Input: part model. Units: mm. Frame: model coordinates. A direction names the side the tool comes from. Round coordinates to 2 decimals unless told otherwise and drop trailing zeros. Order: outer loops, then holes, each group sorted by start corner. A loop starts at its lowest first (then second) coordinate and runs counter-clockwise, first axis right, second up. Notation, with made-up numbers: (30.25, -9.75) -> (60.25, -9.75) arc R13 cw to (60.25, 5.25) -> close; hole circle Ø3 at (83, 24.25). An arc over 180 degrees is marked (long way). Use a Markdown table: item, result.
from build123d import *

# Parameters (mm, degrees)
REVOLVE1_ANGLE      = 180
SKETCH4_R           = 41.29501491
BOSS_EXTRUDE1_DEPTH = 7
SKETCH5_R           = 34.5
BOSS_EXTRUDE2_DEPTH = 12
SKETCH6_R           = 39
BOSS_EXTRUDE4_DEPTH = 4
SKETCH7_R           = 30
CUT_EXTRUDE1_DEPTH  = 24
CUT_EXTRUDE2_DEPTH  = 10


with BuildPart() as part:
    # Sketch1 → Revolve1 (revolve)
    with BuildSketch(Plane(origin=(0, 0, 0), x_dir=(1, 0, 0), z_dir=(0, 1, 0))):
        with BuildLine():
            Line((1.220496419, 44.983445716), (-1.220496419, -44.983445716))
            ThreePointArc((-1.220496419, -44.983445716), (44.983445716, -1.220496419), (1.220496419, 44.983445716))
        make_face()
    revolve(axis=Axis((1.220496419, 0, -44.983445716), (-0.027122143, 0, 0.999632127)), revolution_arc=REVOLVE1_ANGLE)

    # Sketch2 → Cut-Revolve1 (revolve, cut)
    with BuildSketch(Plane.XZ):
        with BuildLine():
            Line((39.984553657, 1.111516454), (-39.984553657, -1.111516454))
            ThreePointArc((-39.984553657, -1.111516454), (-1.111516454, 39.984553657), (39.984553657, 1.111516454))
        make_face()
    revolve(axis=Axis((39.984553657, 0, 1.111516454), (-0.999613841, 0, -0.027787911)), mode=Mode.SUBTRACT)

    # Sketch4 → Boss-Extrude1 (add)
    with BuildSketch(Plane.XZ):
        Circle(SKETCH4_R)
    extrude(amount=-BOSS_EXTRUDE1_DEPTH)

    # Sketch5 → Boss-Extrude2 (add)
    with BuildSketch(Plane.XZ):
        Circle(SKETCH5_R)
    extrude(amount=BOSS_EXTRUDE2_DEPTH)

    # Sketch6 → Boss-Extrude4 (add)
    with BuildSketch(Plane.XZ.offset(12)):
        Circle(SKETCH6_R)
    extrude(amount=-BOSS_EXTRUDE4_DEPTH)

    # Sketch7 → Cut-Extrude1 (cut)
    with BuildSketch(Plane.XZ.offset(12)):
        Circle(SKETCH7_R)
    extrude(amount=-CUT_EXTRUDE1_DEPTH, mode=Mode.SUBTRACT)

    # Sketch8 → Cut-Extrude2 (cut)
    with BuildSketch(Plane.XZ.offset(12)):
        with BuildLine():
            ThreePointArc((37.671107225, 10.093942759), (19.5, 33.774990748), (-10.093942759, 37.671107225))
            Line((-10.093942759, 37.671107225), (-9.058666579, 33.80740392))
            ThreePointArc((-9.058666579, 33.80740392), (17.5, 30.310889132), (33.80740392, 9.058666579))
            Line((33.80740392, 9.058666579), (37.671107225, 10.093942759))
        make_face()
        with BuildLine():
            ThreePointArc((-10.093942759, -37.671107225), (19.5, -33.774990748), (37.671107225, -10.093942759))
            Line((37.671107225, -10.093942759), (33.80740392, -9.058666579))
            ThreePointArc((33.80740392, -9.058666579), (17.5, -30.310889132), (-9.058666579, -33.80740392))
            Line((-9.058666579, -33.80740392), (-10.093942759, -37.671107225))
        make_face()
        with BuildLine():
            Line((-24.748737342, 24.748737342), (-27.577164466, 27.577164466))
            ThreePointArc((-27.577164466, 27.577164466), (-39, 0), (-27.577164466, -27.577164466))
            Line((-27.577164466, -27.577164466), (-24.748737342, -24.748737342))
            ThreePointArc((-24.748737342, -24.748737342), (-35, 0), (-24.748737342, 24.748737342))
        make_face()
    extrude(amount=-CUT_EXTRUDE2_DEPTH, mode=Mode.SUBTRACT)


solid = part.part
1) Cut plane C-C on y = 5.5. Return loops of the section in (x, z).
Answer key:
| item | result |
|---|---|
| outline | circle Ø89.33 at (0, 0); hole circle Ø60 at (0, 0) |
2) Cut plane D-D on y = 22. Return loops of the section in (x, z), and give its area (3 significant figures).
Answer key:
| item | result |
|---|---|
| outline | circle Ø78.51 at (0, 0); hole circle Ø66.81 at (0, 0) |
| area | 1,340 mm^2 |
3) Cut plane B-B on x = 0. Return loops of the section in (y, z).
Answer key:
| item | result |
|---|---|
| outline | (-12, -35) -> (-8, -35) -> (-8, -34.5) -> (0, -34.5) -> (0, -45) arc R45 ccw to (0, 45) -> (0, 34.5) -> (-8, 34.5) -> (-8, 35) -> (-12, 35) -> (-12, 30) -> (7, 30) -> (7, 39.38) arc R40 cw to (7, -39.38) -> (7, -30) -> (-12, -30) -> close |
4) Draft query along Z for faces 1 (the face through (32.907, -3.944, 10.363)), 2 (the face through (-19.624, -10.028, -33.703)), 3 (the face through (-26, -10, -26)). Return one class per face: released by +Z, released by -Z, zero draft, split by the parting line, or undercut.
Answer key:
| item | result |
|---|---|
| face 1 | split by the parting line |
| face 2 | released by -Z |
| face 3 | undercut |
5) Ray query, probe 1 along Z at (x, y) = (0, -6); probe 2 along Y at (x, z) = (-10, -35); probe 3 along Z at (x, y) = (0, 0.5). Return the intervals inside material, ascending.
Answer key:
| item | result |
|---|---|
| probe 1 | z = -34.5 to -30, 30 to 34.5 |
| probe 2 | y = -12 to -8, 0 to 7, 16.58 to 26.46 |
| probe 3 | z = -45 to -30, 30 to 45 |
6) Cut plane A-A on z = 0. Return loops of the section in (x, y), and give its area (3 significant figures).
Answer key:
| item | result |
|---|---|
| outline | (-45, 0) -> (-34.5, 0) -> (-34.5, -8) -> (-35, -8) -> (-35, -12) -> (-30, -12) -> (-30, 7) -> (-39.38, 7) arc R40 cw to (39.38, 7) -> (30, 7) -> (30, -12) -> (39, -12) -> (39, -8) -> (34.5, -8) -> (34.5, 0) -> (45, 0) arc R45 ccw to start |
| area | 933 mm^2 |
7) Contact query for flat-ended pins moving along their axis: P1, Ø5, axis at y = 20, z = 4, coming from the -X side; P2, Ø3, axis at y = 16.5, z = -12, coming from the -X side; P3, Ø4, axis at y = 8, z = -18, coming from the -X side. Output: stop coordinate, or through.
Answer key:
| item | result |
|---|---|
| P1 | stops at x = -41.29 |
| P2 | stops at x = -40.84 |
| P3 | stops at x = -41.37 |
8) Set-up query: faces 4 (the face through (-9.584, -10.028, 35.766)), 5 (the face through (-9.57, -10.03, -35.71)), 6 (the face through (-19.376, -10.028, 33.846)). Return all of +Z, -Z, +X, -X, +Y, -Y with unobstructed straight access to the full face (end or side cutting, diameter ignored); none if empty.
Answer key:
| item | result |
|---|---|
| face 4 | +Z, -Y |
| face 5 | -Z, -Y |
| face 6 | +Z, -X, -Y |
